Model file for the job. Use its own axes, mm. Round coordinates to 2 decimals unless told otherwise and drop trailing zeros. Loops run counter-clockwise (first coordinate to the right, second up) from the corner with the lowest first, then second, coordinate; pieces in that order, holes last.
from build123d import *

# Parameters (mm, degrees)
SKETCH1_R           = 2
SKETCH1_R_2         = 4.5
BOSS_EXTRUDE1_DEPTH = 10


with BuildPart() as part:
    # Sketch1 → Boss-Extrude1 (new body)
    with BuildSketch(Plane.XY):
        with BuildLine():
            Line((0, 0), (360, 0))
            Line((360, 0), (360, -45))
            Line((360, -45), (340, -45))
            Line((340, -45), (340, -40))
            ThreePointArc((340, -40), (339.121320344, -37.878679656), (337, -37))
            Line((337, -37), (23, -37))
            ThreePointArc((23, -37), (20.878679656, -37.878679656), (20, -40))
            Line((20, -40), (20, -45))
            Line((20, -45), (0, -45))
            Line((0, -45), (0, 0))
        make_face()
        with Locations((350, -10)):
            Circle(SKETCH1_R, mode=Mode.SUBTRACT)
        with Locations((350, -30)):
            Circle(SKETCH1_R, mode=Mode.SUBTRACT)
        with Locations((10, -10)):
            Circle(SKETCH1_R, mode=Mode.SUBTRACT)
        with Locations((10, -30.004476127)):
            Circle(SKETCH1_R, mode=Mode.SUBTRACT)
        with Locations((180, -18.5)):
            Circle(SKETCH1_R_2, mode=Mode.SUBTRACT)
        with Locations((255, -18.5)):
            Circle(SKETCH1_R_2, mode=Mode.SUBTRACT)
        with Locations((105, -18.5)):
            Circle(SKETCH1_R_2, mode=Mode.SUBTRACT)
    extrude(amount=BOSS_EXTRUDE1_DEPTH)


solid = part.part
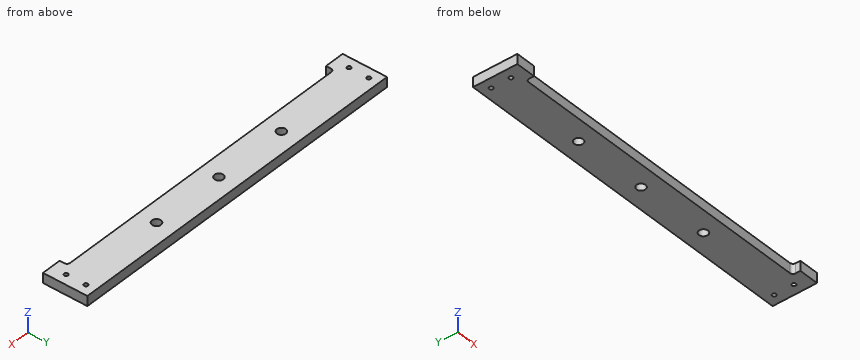
Q1. Probe line 1 (Y direction, x = 350, z = 7.25); line 2 (Y direction, x = 255, z = 5.75); line 3 (X direction, y = -40, z = 9.5). List the from-to ranges inside material, lowest first.
Q2. Slice it at A-A on x = 105. Give the cut face in (y, z), plus the area to 3 significant figures.
Q3. Slice it at B-B on y = -18.5. Give the cut face in (x, z).
Q4. Slice it at C-C on z = 3.25. Give the cut face in (x, y), plus the area to 3 significant figures.
Q5. Flat gauge pins, fed straight in: P1, Ø3, axis at x = 220.5, z = 4.5, coming from the -Y side; P2, Ø2.5, axis at x = 350, y = -30, coming from the +Z side. Where does each tip first touch, or does it go through?
Reply:
1. line 1: y = -45 to -32, -28 to -12, -8 to 0
1. line 2: y = -37 to -23, -14 to 0
1. line 3: x = 0 to 20, 340 to 360
2. outline: (-37, 0) - (-23, 0) - (-23, 10) - (-37, 10) - close; (-14, 0) - (0, 0) - (0, 10) - (-14, 10) - close
2. area: 280 mm2
3. outline: (0, 0) - (100.5, 0) - (100.5, 10) - (0, 10) - close; (109.5, 0) - (175.5, 0) - (175.5, 10) - (109.5, 10) - close; (184.5, 0) - (250.5, 0) - (250.5, 10) - (184.5, 10) - close; (259.5, 0) - (360, 0) - (360, 10) - (259.5, 10) - close
4. outline: (0, -45) - (20, -45) - (20, -40) arc R3 cw to (23, -37) - (337, -37) arc R3 cw to (340, -40) - (340, -45) - (360, -45) - (360, 0) - (0, 0) - close; hole circle Ø4 at (10, -30); hole circle Ø4 at (10, -10); hole circle Ø9 at (105, -18.5); hole circle Ø9 at (180, -18.5); hole circle Ø9 at (255, -18.5); hole circle Ø4 at (350, -30); hole circle Ø4 at (350, -10)
4. area: 13,400 mm2
5. P1: stops at y = -37
5. P2: passes through
